from build123d import *

# Parameters (mm, degrees)
SKETCH_W     = 56
SKETCH_H     = 42
PAD_DEPTH    = 10
SKETCH002_W  = 50
SKETCH002_H  = 36
POCKET_DEPTH = 8
FILLET_R     = 1
FILLET001_R  = 1
FILLET002_R  = 1
FILLET003_R  = 1
SKETCH003_R  = 3
HOLE_DEPTH   = 25


with BuildPart() as part:
    # Sketch → Pad (new body)
    with BuildSketch(Plane.XY):
        Rectangle(SKETCH_W, SKETCH_H)
    extrude(amount=PAD_DEPTH)

    # Sketch002 (on Face6 of Pad) → Pocket (cut)
    with BuildSketch(Plane.XY.offset(10)):
        Rectangle(SKETCH002_W, SKETCH002_H)
    extrude(amount=-POCKET_DEPTH, mode=Mode.SUBTRACT)

    # Fillet
    fillet_edges = [part.edges().sort_by_distance(p)[0] for p in [
        (-25, 18, 6),
    ]]
    fillet(fillet_edges, radius=FILLET_R)

    # Fillet001
    fillet001_edges = [part.edges().sort_by_distance(p)[0] for p in [
        (25, 18, 6),
    ]]
    fillet(fillet001_edges, radius=FILLET001_R)

    # Fillet002
    fillet002_edges = [part.edges().sort_by_distance(p)[0] for p in [
        (25, -18, 6),
    ]]
    fillet(fillet002_edges, radius=FILLET002_R)

    # Fillet003
    fillet003_edges = [part.edges().sort_by_distance(p)[0] for p in [
        (-25, -18, 6),
    ]]
    fillet(fillet003_edges, radius=FILLET003_R)

    # Sketch003 (on Face14 of Fillet003) → Hole (cut)
    with BuildSketch(Plane.XY.offset(2)):
        with Locations((-14, 8.6)):
            Circle(SKETCH003_R)
        with Locations((14, -8.6)):
            Circle(SKETCH003_R)
    extrude(amount=-HOLE_DEPTH, mode=Mode.SUBTRACT)


solid = part.part
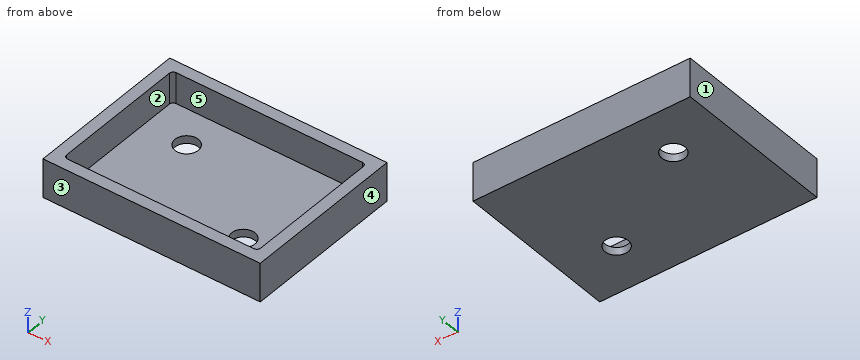
Work out the finished part from the listing and answer in its coordinate system (mm). Face numbers are marked on the shaded views. A direction names the side the tool comes from. Round coordinates to 2 decimals unless told otherwise and drop trailing zeros. Write each loop counter-clockwise with the first axis right and the second up, starting at its lowest first coordinate (ties: lowest second). Pieces come first, ordered by that corner, then holes. Notation, with made-up numbers: (-19.75, -23) -> (19.25, -23) arc R27 ccw to (19.25, 12) -> close; hole circle Ø6 at (-38, 51.5). An arc over 180 degrees is marked (long way). Write each question's results on one line, items separated by ' | '.
Item 1: Find the intervals of material crossed by line 1 along X through (y, z) = (-4, 5.75); line 2 along Y through (x, z) = (-21.5, 5.5); line 3 along Y through (x, z) = (14, 0.85), in increasing order. Write a range as [from, to].
Result set:
line 1: [-28, -25], [25, 28] | line 2: [-21, -18], [18, 21] | line 3: [-21, -11.6], [-5.6, 21]
Item 2: A cutting plane is placed at A-A, the plane y = 11. Determine the outline of the cut face in (x, z).
Result set:
outline: (-28, 0) -> (-15.8, 0) -> (-15.8, 2) -> (-25, 2) -> (-25, 10) -> (-28, 10) -> close; (-12.2, 0) -> (28, 0) -> (28, 10) -> (25, 10) -> (25, 2) -> (-12.2, 2) -> close
Item 3: A cutting plane is placed at D-D, the plane x = 5.5. Determine the outline of the cut face in (y, z), plus the area to 3 significant figures.
Result set:
outline: (-21, 0) -> (21, 0) -> (21, 10) -> (18, 10) -> (18, 2) -> (-18, 2) -> (-18, 10) -> (-21, 10) -> close | area: 132 mm^2
Item 4: A cutting plane is placed at C-C, the plane z = 7.75. Determine the outline of the cut face in (x, y), plus the area to 3 significant figures.
Result set:
outline: (-28, -21) -> (28, -21) -> (28, 21) -> (-28, 21) -> close; hole (-25, -17) arc R1 ccw to (-24, -18) -> (24, -18) arc R1 ccw to (25, -17) -> (25, 17) arc R1 ccw to (24, 18) -> (-24, 18) arc R1 ccw to (-25, 17) -> close | area: 553 mm^2
Item 5: Which of the six approach directions +Z, -Z, +X, -X, +Y, -Y give full straight-line access (tool end or side, diameter ignored) to the marked faces 1 and 2?
Result set:
face 1: +Z, -Z, -X, +Y, -Y | face 2: +Z
Item 6: The mould has two halves that part along Y. Classify the marked faces 3, 4 and 5: +Y half, -Y half, draft (parallel to the pull), parting line (faces both ways), or undercut.
Result set:
face 3: -Y half | face 4: draft | face 5: undercut
Item 7: A cutting plane is placed at B-B, the plane x = -14. Determine the outline of the cut face in (y, z), plus the area to 3 significant figures.
Result set:
outline: (-21, 0) -> (5.6, 0) -> (5.6, 2) -> (-18, 2) -> (-18, 10) -> (-21, 10) -> close; (11.6, 0) -> (21, 0) -> (21, 10) -> (18, 10) -> (18, 2) -> (11.6, 2) -> close | area: 120 mm^2
Item 8: Flat-ended cylindrical pins translate along their axes: P1, Ø12, axis at x = 8.5, y = 5.5, coming from the +Z side; P2, Ø5, axis at x = 2, y = 5.5, coming from the -Z side. Find the tip coordinate at first contact, or state that the pin passes through.
Result set:
P1: z = 2 | P2: z = 0
